Could you check a few things on this model? Use its own coordinates, in mm. A direction names the side the tool comes from. Round coordinates to 2 decimals unless told otherwise and drop trailing zeros. Order: outer loops, then holes, each group sorted by start corner. A loop starts at its lowest first (then second) coordinate and runs counter-clockwise, first axis right, second up. Notation, with made-up numbers: (59, 60.5) - (107, 60.5) arc R24 cw to (107, 82.5) - close; hole circle Ø7 at (4.5, 50). An arc over 180 degrees is marked (long way). Use one line per item in the form item = value.
Autodesk Inventor part; units mm, degrees
ref_plane "YZ Plane" through (0, 0, 0) normal (1, 0, 0) x (0, 1, 0)
ref_plane "XZ Plane" through (0, 0, 0) normal (0, 1, 0) x (-1, 0, 0)
ref_plane "XY Plane" through (0, 0, 0) normal (0, 0, 1) x (1, 0, 0)
sketch "Эскиз1" plane through (0, 0, 0) normal (1, 0, 0) x (0, 1, 0)
  line L0 (0.3766, -35.0912) -> (12.3766, -35.0912)
  line L1 (12.3766, -35.0912) -> (12.3766, -47.0912)
  line L2 (12.3766, -47.0912) -> (28.3766, -47.0912)
  line L3 (28.3766, -32.0912) -> (50.3766, -32.0912)
  line L4 (50.3766, -32.0912) -> (50.3766, -24.0912)
  line L5 (50.3766, -24.0912) -> (30.3766, -24.0912)
  line L6 (30.3766, -24.0912) -> (30.3766, -13.0912)
  line L7 (28.3766, -47.0912) -> (28.3766, -32.0912)
  line L8 (0.3766, -35.0912) -> (0.3766, -27.0912)
  line L9 (0.3766, -27.0912) -> (8.3766, -27.0912)
  line L10 (8.3766, -27.0912) -> (8.3766, -19.0912)
  line L11 (8.3766, -19.0912) -> (0.3766, -19.0912)
  line L12 (0.3766, -19.0912) -> (0.3766, -13.0912)
  line L13 (0.3766, -13.0912) -> (30.3766, -13.0912)
  point P0 (0, 0)
  point P1 (-47.0655, -24.8908)
extrude "Выдавливание1" add sketch "Эскиз1" along normal blind 10
equation "\"Радиус_гибки\" = Толщина"
equation "\"Ширина_просечки\" = Толщина"
equation "\"Глубина_просечки\" = 0.5 * Толщина"
equation "\"Размер_просечки\" = 4 * Толщина"
equation "\"Мин_остаток\" = 2 * Толщина"
equation "\"Радиус_перехода\" = Радиус_гибки"
equation "\"Радиус_Якоби\" = Радиус_гибки"
equation "\"Размер_зазора\" = Толщина"
Item 1: Will these pins go through, and if not, where does the flat tip stop? P1, Ø10, axis at y = 8, z = -42, coming from the +X side; P2, Ø5, axis at x = 2.5, y = 38.5, coming from the +Z side; P3, Ø1.5, axis at x = 7.5, z = -41, coming from the +Y side; P4, Ø6, axis at x = 5, z = -18, coming from the +Y side.
Found:
P1 = 10
P2 = -24.09
P3 = 28.38
P4 = 30.38
Item 2: If we mould it in two halves opening along Z, with no side actions, what happens to faces 1 (the face through (5, 41, -24.091)), 2 (the face through (10, 19, -30)), 3 (the face through (5, 4, -19.091))? For each: released by +Z, released by -Z, zero draft, split by the parting line, or undercut.
Found:
face_1 = released by +Z
face_2 = zero draft
face_3 = undercut
Item 3: Imagine slicing it at C-C on y = 29.5. Please give me the cut outline in (x, z), plus the area to 3 significant figures.
Found:
outline = (0, -32.09) - (10, -32.09) - (10, -13.09) - (0, -13.09) - close
area = 190 mm2
Item 4: For faces 4 (the face through (5, 28.377, -40)), 5 (the face through (5, 12.377, -41)), 6 (the face through (5, 4, -27.091)), which set-ups out of +Z, -Z, +X, -X, +Y, -Y let a thin tool reach every point of the face, with its end or its side?
Found:
face_4 = -Z, +X, -X, +Y
face_5 = -Z, +X, -X, -Y
face_6 = +X, -X, -Y
Item 5: I need wall thicknesses on L1, parallel to Z at x = 8.25, y = 41.5; L2, parallel to Y at x = 1.25, z = -37; L3, parallel to Y at x = 4.75, z = -35. Which ranges of each line are inside material? Lowest first, please.
Found:
L1 = -32.09 to -24.09
L2 = 12.38 to 28.38
L3 = 0.38 to 28.38
Item 6: Imagine slicing it at A-A on x = 1.75. Please give me the cut outline in (y, z).
Found:
outline = (0.38, -35.09) - (12.38, -35.09) - (12.38, -47.09) - (28.38, -47.09) - (28.38, -32.09) - (50.38, -32.09) - (50.38, -24.09) - (30.38, -24.09) - (30.38, -13.09) - (0.38, -13.09) - (0.38, -19.09) - (8.38, -19.09) - (8.38, -27.09) - (0.38, -27.09) - close
Item 7: Imagine slicing it at B-B on z = -43. Please give me the cut outline in (x, y), plus the area to 3 significant figures.
Found:
outline = (0, 12.38) - (10, 12.38) - (10, 28.38) - (0, 28.38) - close
area = 160 mm2
